Here's how the part is built. I have some questions about the finished solid (model axes, mm). Face numbers are marked on the shaded views. A direction names the side the tool comes from. Round coordinates to 2 decimals unless told otherwise and drop trailing zeros. Write each loop counter-clockwise with the first axis right and the second up, starting at its lowest first coordinate (ties: lowest second). Pieces come first, ordered by that corner, then holes. Notation, with made-up numbers: (41.5, 64) - (62.5, 64) arc R33 cw to (62.5, 100) - close; hole circle Ø9 at (-39, 79.5). An arc over 180 degrees is marked (long way). Write item = value, one per line. Start each with the question number.
Item 1: If I drill on line 1 along Z through (x, y) = (-16, 17); line 2 along Y through (x, z) = (-4, 60); line 3 along Y through (x, z) = (-5, 35), over which ranges is the centre line in solid material (lowest first)? Write a range as [from, to].
Item 2: If we section it at B-B (y = 45.5): Please give me the cut outline in (x, z), and give its area (3 significant figures).
Item 3: Thinking about a two-plate mould opening in Y: for the marked faces 1, 2, 3 and 4, which applies, pulls with the +Y half, pulls with the -Y half, needs draft (parallel to the pull), parting line crosses it, or undercut?
Item 4: If we section it at A-A (x = -6): Please give me the cut outline in (y, z).
Item 5: For P1, Ø14, axis at y = 41.5, z = 31.5, coming from the -X side; P2, Ø3, axis at x = -7.5, y = 8, coming from the -Z side; P3, Ø2.5, axis at x = -4, z = 59, coming from the +Y side; P4, Ø12, axis at x = -21.5, z = 19.5, coming from the +Y side, each with a flat end and sliding along its axis, tell me the tip position at first contact or that it passes through.
Item 6: Which directions (+Z, -Z, +X, -X, +Y, -Y) give clear straight access to the entire face, cutting with the end or side of a thin tool? Please do the marked faces 5, 6, 7, 8 and 9.
```python
from build123d import *
from build123d.topology import SkipClean

# Parameters (mm, degrees)
RESSALTO_EXTRUS_O1_DEPTH = 70
CORTE_EXTRUS_O1_REACH    = 94.871
ESBO_O2_R                = 3.1
FILETE1_DEPTH            = 70
FILETE1_START            = -22
FILETE1_2_OUTLINE_R      = 3.1
FILETE1_2_DEPTH          = 14
ESBO_O3_R                = 5.25
RESSALTO_EXTRUS_O2_DEPTH = 8
CORTE_EXTRUS_O6_DEPTH    = 16


with BuildPart() as part:
    # Esboço1 → Ressalto-extrusão1 (new body)
    with BuildSketch(Plane.XY):
        Polygon((0, 0), (0, 35), (-8, 35), (-8, 8), (-50, 8), (-50, 0), align=None)
    extrude(amount=RESSALTO_EXTRUS_O1_DEPTH)

    # Esboço2 → Corte-extrusão1 (cut, up to next)
    with BuildSketch(Plane(origin=(0, 0, 0), x_dir=(0, 0, -1), z_dir=(1, 0, 0)), mode=Mode.PRIVATE) as corte_extrus_o1_sk1:
        with Locations((-60, 20.050946568)):
            Circle(ESBO_O2_R)
    corte_extrus_o1_tool1 = extrude(corte_extrus_o1_sk1.sketch, amount=-CORTE_EXTRUS_O1_REACH, mode=Mode.PRIVATE) & part.part
    # Esboço2 → Corte-extrusão1 (cut, up to next)
    with BuildSketch(Plane(origin=(0, 0, 0), x_dir=(0, 0, -1), z_dir=(1, 0, 0)), mode=Mode.PRIVATE) as corte_extrus_o1_sk2:
        with Locations((-10, 20.050946568)):
            Circle(ESBO_O2_R)
    corte_extrus_o1_tool2 = extrude(corte_extrus_o1_sk2.sketch, amount=-CORTE_EXTRUS_O1_REACH, mode=Mode.PRIVATE) & part.part
    add(corte_extrus_o1_tool1.solids().sort_by_distance((0, 20.050947, 60))[0], mode=Mode.SUBTRACT)
    add(corte_extrus_o1_tool2.solids().sort_by_distance((0, 20.050947, 10))[0], mode=Mode.SUBTRACT)

    # Filete1: read off the stored shape, not the designer's step
    # Filete1 outline → Filete1 (add)
    with BuildSketch(Plane.XY):
        with BuildLine():
            Line((-8, 8), (-8, 35))
            add(Edge.make_bspline(
                [(-8, 35), (-9.46726927, 11.949085531), (-50, 8)],
                knots=[0, 0, 0, 1, 1, 1], degree=2, weights=[1, 0.761577311, 1]))
            Line((-50, 8), (-8, 8))
        make_face()
    extrude(amount=FILETE1_DEPTH)

    # Filete1 2 outline → Filete1 2 (cut)
    with SkipClean():  # the faces are left unmerged after this step: merging them gives an invalid solid
        with BuildSketch(Plane.YZ.offset(FILETE1_START)):
            with Locations((20.050946568, 10)):
                Circle(FILETE1_2_OUTLINE_R)
            with Locations((20.050946568, 60)):
                Circle(FILETE1_2_OUTLINE_R)
        extrude(amount=FILETE1_2_DEPTH, mode=Mode.SUBTRACT)

    # Esboço3 → Ressalto-extrusão2 (add)
    with SkipClean():  # the faces are left unmerged after this step: merging them gives an invalid solid
        with BuildSketch(Plane(origin=(0, 0, 0), x_dir=(0, 0, -1), z_dir=(1, 0, 0))):
            with BuildLine():
                Line((-52.5, 35), (-17.5, 35))
                ThreePointArc((-17.5, 35), (-22.803300859, 37.196699141), (-25, 42.5))
                ThreePointArc((-25, 42.5), (-35, 52.5), (-45, 42.5))
                ThreePointArc((-45, 42.5), (-47.196699141, 37.196699141), (-52.5, 35))
            make_face()
            with Locations((-35, 42.5)):
                Circle(ESBO_O3_R, mode=Mode.SUBTRACT)
        extrude(amount=-RESSALTO_EXTRUS_O2_DEPTH)

    # Esboço6 → Corte-extrusão6 (cut)
    with BuildSketch(Plane.ZY.offset(8)):
        Polygon((4, 23.515048183), (4, 16.586844953), (10, 13.122743338), (16, 16.586844953), (16, 23.515048183), (10, 26.979149798), align=None)
        Polygon((54, 23.515048183), (54, 16.586844953), (60, 13.122743338), (66, 16.586844953), (66, 23.515048183), (60, 26.979149798), align=None)
    extrude(amount=CORTE_EXTRUS_O6_DEPTH, mode=Mode.SUBTRACT)


solid = part.part
```
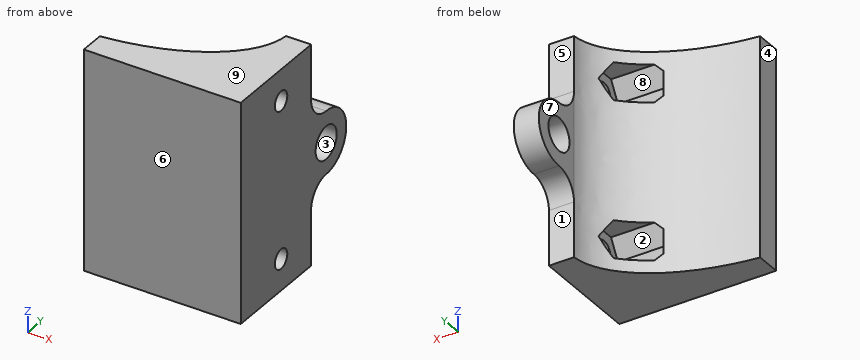
Reply:
q1.line_1 = [0, 4], [16, 54], [66, 70]
q1.line_2 = [0, 16.95], [23.15, 35]
q1.line_3 = [0, 37.25], [47.75, 52.5]
q2.outline = (-8, 25.46) - (0, 25.46) - (0, 30.69) - (-8, 30.69) - close; (-8, 39.31) - (0, 39.31) - (0, 44.54) - (-8, 44.54) - close
q2.area = 83.7 mm2
q3.face_1 = pulls with the +Y half
q3.face_2 = undercut
q3.face_3 = undercut
q3.face_4 = needs draft
q4.outline = (0, 0) - (35, 0) - (35, 17.5) arc R7.5 cw to (42.5, 25) arc R10 ccw to (42.5, 45) arc R7.5 cw to (35, 52.5) - (35, 70) - (0, 70) - close; hole circle Ø6.2 at (20.05, 10); hole circle Ø6.2 at (20.05, 60); hole circle Ø10.5 at (42.5, 35)
q5.P1 = -8.04
q5.P2 = 0
q5.P3 = 35
q5.P4 = 21.22
q6.face_5 = +Z, +X, -X, +Y
q6.face_6 = +Z, -Z, +X, -X, -Y
q6.face_7 = +Z, -Z, -X, +Y
q6.face_8 = none
q6.face_9 = +Z, +X, -X, +Y, -Y
